Could you check a few things on this model? Use its own coordinates, in mm. Give positions to 0.01 mm unless a question says otherwise; leave off trailing zeros. Order: outer loops, then holes, each group sorted by start corner. A loop starts at its lowest first (then second) coordinate and runs counter-clockwise, first axis right, second up.
(1) If I drill on probe 1 along Y at (x, z) = (0.25, 91.5); probe 2 along X at (y, z) = (-0.5, 106.5); probe 3 along X at (y, z) = (1, 70.5), over which ranges is the centre line in solid material (lowest first)?
(2) Imagine slicing it at A-A, the plane y = 0. Write out the boundary of the cut face in (x, z), then the cut area to 3 significant figures.
(3) Imagine slicing it at C-C, the plane z = 133. Write out the boundary of the cut face in (x, y), then the cut area to 3 significant figures.
(4) If we mould it in two halves opening along X, with no side actions, what happens to faces 1 (the cylindrical face through (-0.867, -3.905, 123.25)), 2 (the flat face through (5, 0, 235)), 3 (the flat face through (-5, 0, 247)), 4 (the flat face through (0, 5, 123))? For each: released by +X, released by -X, zero draft, split by the parting line, or undercut.
(5) Imagine slicing it at B-B, the plane x = 0. Write out the boundary of the cut face in (y, z).
from build123d import *

# Parameters (mm, degrees)
SKETCH1_W           = 10
SKETCH1_H           = 10
SKETCH1_R           = 4
BOSS_EXTRUDE1_DEPTH = 250
SKETCH2_R           = 1.6
CUT_EXTRUDE1_DEPTH  = 11


with BuildPart() as part:
    # Sketch1 → Boss-Extrude1 (new body)
    with BuildSketch(Plane.XY):
        Rectangle(SKETCH1_W, SKETCH1_H)
        Circle(SKETCH1_R, mode=Mode.SUBTRACT)
    extrude(amount=BOSS_EXTRUDE1_DEPTH)

    # Sketch2 → Cut-Extrude1 (cut, through all)
    with BuildSketch(Plane.XZ.offset(5)):
        with Locations((-6.119289585, 243.266656382)):
            Circle(SKETCH2_R)
        with Locations((6.119289585, 228.733343618)):
            Circle(SKETCH2_R)
        with Locations((-6.119289585, 230.846914034)):
            Circle(SKETCH2_R)
        with Locations((6.119289585, 241.153085966)):
            Circle(SKETCH2_R)
    extrude(amount=-CUT_EXTRUDE1_DEPTH, mode=Mode.SUBTRACT)


solid = part.part
Answer block:
1. probe 1: y = -5 to -3.99, 3.99 to 5
1. probe 2: x = -5 to -3.97, 3.97 to 5
1. probe 3: x = -5 to -3.87, 3.87 to 5
2. outline: (-5, 0) - (-4, 0) - (-4, 250) - (-5, 250) - (-5, 244.41) arc R1.6 cw to (-5, 242.12) - (-5, 231.99) arc R1.6 cw to (-5, 229.7) - close; (4, 0) - (5, 0) - (5, 227.59) arc R1.6 cw to (5, 229.88) - (5, 240.01) arc R1.6 cw to (5, 242.3) - (5, 250) - (4, 250) - close
2. area: 497 mm2
3. outline: (-5, -5) - (5, -5) - (5, 5) - (-5, 5) - close; hole circle Ø8 at (0, 0)
3. area: 49.7 mm2
4. face 1: undercut
4. face 2: released by +X
4. face 3: released by -X
4. face 4: zero draft
5. outline: (-5, 0) - (-4, 0) - (-4, 250) - (-5, 250) - close; (4, 0) - (5, 0) - (5, 250) - (4, 250) - close
